```python
from build123d import *

# Parameters (mm, degrees)
SKETCH_W             = 47.4
SKETCH_H             = 13
SKETCH_R             = 1.65
PAD_DEPTH            = 10
SKETCH001_R          = 3.75
POCKET_DEPTH         = 5.5
SKETCH002_W          = 12
SKETCH002_H          = 10
POCKET001_DEPTH      = 100
POCKET001_DEPTH_BACK = -2.75
SKETCH003_R          = 1.65
POCKET002_DEPTH      = 5.501
POCKET002_DEPTH_BACK = -7.501
POCKET003_DEPTH      = 5.501
POCKET003_DEPTH_BACK = -7.501
POCKET004_DEPTH      = 2.501


with BuildPart() as part:
    # Sketch → Pad (new body)
    with BuildSketch(Plane.XY):
        with Locations((0, -1)):
            Rectangle(SKETCH_W, SKETCH_H)
        with Locations((-20.5, 0)):
            Circle(SKETCH_R, mode=Mode.SUBTRACT)
        with Locations((20.5, 0)):
            Circle(SKETCH_R, mode=Mode.SUBTRACT)
    extrude(amount=-PAD_DEPTH)

    # Sketch001 → Pocket (cut)
    with BuildSketch(Plane.XY):
        with Locations((-20.481411, -0.058129)):
            Circle(SKETCH001_R)
        with Locations((20.5, 0)):
            Circle(SKETCH001_R)
    extrude(amount=-POCKET_DEPTH, mode=Mode.SUBTRACT)

    # Sketch002 → Pocket001 (cut, two sides)
    with BuildSketch(Plane.XZ) as pocket001_sk:
        with Locations((-6.6, -5)):
            Rectangle(SKETCH002_W, SKETCH002_H)
        with Locations((6.6, -5)):
            Rectangle(SKETCH002_W, SKETCH002_H)
    extrude(amount=-POCKET001_DEPTH, mode=Mode.SUBTRACT)
    extrude(pocket001_sk.sketch, amount=-POCKET001_DEPTH_BACK, mode=Mode.SUBTRACT)

    # Sketch003 → Pocket002 (cut, two sides)
    with BuildSketch(Plane.XZ) as pocket002_sk:
        with Locations((-14.75, -5)):
            Circle(SKETCH003_R)
        with Locations((14.75, -5)):
            Circle(SKETCH003_R)
    extrude(amount=-POCKET002_DEPTH, mode=Mode.SUBTRACT)
    extrude(pocket002_sk.sketch, amount=-POCKET002_DEPTH_BACK, mode=Mode.SUBTRACT)

    # Sketch004 → Pocket003 (cut, two sides)
    with BuildSketch(Plane.XZ) as pocket003_sk:
        Polygon((-18.2, 0), (-23.7, -5.5), (-23.7, 0), align=None)
        Polygon((18.2, 0), (23.7, 0), (23.7, -5.5), align=None)
    extrude(amount=-POCKET003_DEPTH, mode=Mode.SUBTRACT)
    extrude(pocket003_sk.sketch, amount=-POCKET003_DEPTH_BACK, mode=Mode.SUBTRACT)

    # Sketch005 (on DatumPlane) → Pocket004 (cut, through all)
    with BuildSketch(Plane.XZ.offset(5)):
        Polygon((-13.090118, -7.875), (-11.430236, -5), (-13.090118, -2.125), (-16.409882, -2.125), (-18.069764, -5), (-16.409882, -7.875), align=None)
        Polygon((16.409882, -7.875), (18.069764, -5), (16.409882, -2.125), (13.090118, -2.125), (11.430236, -5), (13.090118, -7.875), align=None)
    extrude(amount=POCKET004_DEPTH, mode=Mode.SUBTRACT)


solid = part.part
```
Build history of the part. All positions in model axes, mm. A direction names the side the tool comes from. Give positions to 0.01 mm unless a question says otherwise; leave off trailing zeros. Loops run counter-clockwise (first coordinate to the right, second up) from the corner with the lowest first, then second, coordinate; pieces in that order, holes last.
1) 3-axis set-ups, long thin cutter, end or side, ignore diameter. For faces 1 (the face through (-12.6, 1, -5)), 2 (the face through (-16.734, -0.195, -3.323)), 3 (the face through (17.25, -6.23, -3.58)): which of +Z, -Z, +X, -X, +Y, -Y reach the whole face in a straight line?
Values follow:
face 1: +Z, -Z, +Y
face 2: +Z
face 3: -Y
2) Band-saw the part on B-B on x = -14.75. List the corners of the cut face in (y, z) (3 decimals).
Values follow:
outline: (-7.5, -10) - (5.5, -10) - (5.5, -6.65) - (-5, -6.65) - (-5, -7.875) - (-7.5, -7.875) - close; (-7.5, -2.125) - (-5, -2.125) - (-5, -3.35) - (5.5, -3.35) - (5.5, 0) - (-7.5, 0) - close
3) Band-saw the part on D-D on y = -4.5. List the corners of the cut face in (x, z), then the cut area to 3 significant figures.
Values follow:
outline: (-23.7, -10) - (23.7, -10) - (23.7, -5.5) - (18.2, 0) - (-18.2, 0) - (-23.7, -5.5) - close; hole circle Ø3.3 at (-14.75, -5); hole circle Ø3.3 at (14.75, -5)
area: 427 mm2
4) Probe line 1 along X through (y, z) = (-0.25, -0.75); line 2 along X through (y, z) = (3, -6.75); line 3 along Z through (x, y) = (-14.75, -2). List the from-to ranges inside material, lowest first.
Values follow:
line 1: x = -16.74 to -12.6, -0.6 to 0.6, 12.6 to 16.76
line 2: x = -23.7 to -12.6, -0.6 to 0.6, 12.6 to 23.7
line 3: z = -10 to -6.65, -3.35 to 0
5) Drop flat-ended pins along their axis: P1, Ø2, axis at x = 21, y = -0.5, coming from the +Z side; P2, Ø1, axis at y = 2, z = -1, coming from the -X side; P3, Ø3, axis at x = 14.5, z = -4.5, coming from the -Y side. Give the stop position or say it passes through.
Values follow:
P1: stops at z = -5.5
P2: stops at x = -17.74
P3: stops at y = -5
6) Two-plate mould, pull along Y, no slides. Class faces 4 (the face through (-13, -5, -4)), 5 (the face through (18.85, 0.07, -7.72)), 6 (the face through (12.25, -6.23, -6.42)): released by +Y, released by -Y, zero draft, split by the parting line, or undercut.
Values follow:
face 4: released by -Y
face 5: undercut
face 6: zero draft
7) Band-saw the part on A-A on y = 0. List the corners of the cut face in (x, z), then the cut area to 3 significant figures.
Values follow:
outline: (-23.7, -10) - (-22.15, -10) - (-22.15, -5.5) - (-23.7, -5.5) - close; (-18.85, -10) - (-12.6, -10) - (-12.6, 0) - (-16.73, 0) - (-16.73, -5.5) - (-18.85, -5.5) - close; (-0.6, -10) - (0.6, -10) - (0.6, 0) - (-0.6, 0) - close; (12.6, -10) - (18.85, -10) - (18.85, -5.5) - (16.75, -5.5) - (16.75, 0) - (12.6, 0) - close; (22.15, -10) - (23.7, -10) - (23.7, -5.5) - (22.15, -5.5) - close; hole circle Ø3.3 at (-14.75, -5); hole circle Ø3.3 at (14.75, -5)
area: 111 mm2
8) Band-saw the part on C-C on z = -9. List the corners of the cut face in (x, y), then the cut area to 3 significant figures.
Values follow:
outline: (-23.7, -7.5) - (23.7, -7.5) - (23.7, 5.5) - (12.6, 5.5) - (12.6, -2.75) - (0.6, -2.75) - (0.6, 5.5) - (-0.6, 5.5) - (-0.6, -2.75) - (-12.6, -2.75) - (-12.6, 5.5) - (-23.7, 5.5) - close; hole circle Ø3.3 at (-20.5, 0); hole circle Ø3.3 at (20.5, 0)
area: 401 mm2
